from build123d import *

# Parameters (mm, degrees)
ESQUISSE1_R                                   = 5
BOSS_EXTRU_1_DEPTH                            = 90
ESQUISSE2_R                                   = 2.5
BOSS_EXTRU_2_DEPTH                            = 10
TROU_POUR_TARAUDAGE_POUR_TROU_TARAUD_M5_D     = 4.2
TROU_POUR_TARAUDAGE_POUR_TROU_TARAUD_M5_DEPTH = 10
TROU_POUR_TARAUDAGE_POUR_TROU_TARAUD_M5_TIP   = 1.2618073
CHANFREIN1_SIZE                               = 0.5


with BuildPart() as part:
    # Esquisse1 → Boss.-Extru.1 (new body)
    with BuildSketch(Plane.XY):
        Circle(ESQUISSE1_R)
    extrude(amount=BOSS_EXTRU_1_DEPTH)

    # Esquisse2 → Boss.-Extru.2 (add)
    with BuildSketch(Plane(origin=(0, 0, 0), x_dir=(-1, 0, 0), z_dir=(0, 0, -1))):
        Circle(ESQUISSE2_R)
    extrude(amount=BOSS_EXTRU_2_DEPTH)

    # Trou pour taraudage pour trou taraudé M51
    with Locations(Plane.XY.offset(90)):
        with Locations((0, 0)):
            Hole(TROU_POUR_TARAUDAGE_POUR_TROU_TARAUD_M5_D / 2, depth=TROU_POUR_TARAUDAGE_POUR_TROU_TARAUD_M5_DEPTH)
            with Locations((0, 0, -(TROU_POUR_TARAUDAGE_POUR_TROU_TARAUD_M5_DEPTH + TROU_POUR_TARAUDAGE_POUR_TROU_TARAUD_M5_TIP / 2))):  # 118° drill point
                Cone(0, TROU_POUR_TARAUDAGE_POUR_TROU_TARAUD_M5_D / 2, TROU_POUR_TARAUDAGE_POUR_TROU_TARAUD_M5_TIP, mode=Mode.SUBTRACT)

    # Chanfrein1
    chanfrein1_edges = [part.edges().sort_by_distance(p)[0] for p in [
        (-5, 0, 0),
        (-5, 0, 90),
        (2.5, 0, -10),
    ]]
    chamfer(chanfrein1_edges, length=CHANFREIN1_SIZE)


solid = part.part
Read the model definition and answer for the solid it produces. Units are mm, in the model's axes. A direction names the side the tool comes from. Round coordinates to 2 decimals unless told otherwise and drop trailing zeros. Write each loop counter-clockwise with the first axis right and the second up, starting at its lowest first coordinate (ties: lowest second). Pieces come first, ordered by that corner, then holes.
1. Straight lines are drawn through the part: L1, parallel to Y at x = 0, z = 85.5; L2, parallel to Z at x = -3, y = -0.5; L3, parallel to X at y = -2.25, z = 46.5. For each, find the intervals that lie inside material, in ascending order.
2. Which of the six approach directions +Z, -Z, +X, -X, +Y, -Y give full straight-line access (tool end or side, diameter ignored) to faces 4 (the face through (-2.003, 0.631, 84.93)), 5 (the face through (2, -2, 0)), 6 (the face through (-2.1, -0.9, 90))?
3. The part is cut by section A-A, the plane z = 12.5. Determine the outline of the cut face in (x, y).
4. Determine the mould class of faces 1 (the face through (0.54, -2.44, -4.68)), 2 (the face through (0, 0, -10)), 3 (the face through (0.35, 0.11, 78.96)) for opening direction X: pulls with the +X half, pulls with the -X half, needs draft (parallel to the pull), parting line crosses it, or undercut.
5. Given pin 1 Ø1 at (y, z) = (1.5, 55.5) entering from -X; pin 2 Ø1.5 at (y, z) = (2.5, 67) entering from -X; pin 3 Ø3 at (y, z) = (-0.5, 55.5) entering from +X; pin 4 Ø4 at (x, y) = (0, 0) entering from +Z, each flat-ended and moving along its own axis, determine where each tip first touches the part or whether it passes through.
Values:
1. L1: y = -5 to -2.1, 2.1 to 5
1. L2: z = 0 to 90
1. L3: x = -4.47 to 4.47
2. face 4: +Z
2. face 5: -Z
2. face 6: +Z, +X, -X, +Y, -Y
3. outline: circle Ø10 at (0, 0)
4. face 1: parting line crosses it
4. face 2: needs draft
4. face 3: undercut
5. pin 1: stops at x = -4.9
5. pin 2: stops at x = -4.68
5. pin 3: stops at x = 5
5. pin 4: stops at z = 79.94
